The listing builds one solid part. Answer for the finished solid, in the listing's coordinates (mm). A direction names the side the tool comes from. Round coordinates to 2 decimals unless told otherwise and drop trailing zeros. Write each loop counter-clockwise with the first axis right and the second up, starting at its lowest first coordinate (ties: lowest second). Pieces come first, ordered by that corner, then holes.
Item 1: For a pull along Y with two mould halves and no side action, classify faces 1 (the face through (11.01, 6.66, 2.5)), 2 (the face through (6, 2, 4)), 3 (the face through (-3.794, -17.084, 1.479)) as +Y half, -Y half, draft (parallel to the pull), parting line (faces both ways), or undercut.
Item 2: Each of these flat-tipped pins is pushed along its axis until it touches: pin 1 (10.5 mm diameter, centred on x = 12.99, y = -7.5, fed in from +Z); pin 2 (4 mm diameter, centred on y = 3.5, z = 1.5, fed in from +X); pin 3 (6 mm diameter, centred on x = 14, y = -8, fed in from +Z). Where does it stop, or does it pass through?
Item 3: Find section D-D on y = 0. Give the vertices of the cut face in (x, z) (3 decimals).
Item 4: Find the intervals of material crossed by probe 1 along Y at (x, z) = (0, 1); probe 2 along Y at (x, z) = (0, 2.7); probe 3 along Y at (x, z) = (-0.5, 4.75), in increasing order.
Item 5: Find section C-C on z = 5. Give the vertices of the cut face in (x, y) (3 decimals), then the cut area to 3 significant figures.
Item 6: Find section A-A on z = 0.5. Give the vertices of the cut face in (x, y), then the cut area to 3 significant figures.
Item 7: Find section B-B on y = 7.5. Give the vertices of the cut face in (x, z), then the cut area to 3 significant figures.
Item 8: A tool of negligible diameter and unlimited length cuts with its end or side. For faces 4 (the face through (3.476, 0.045, 5.535)), 5 (the face through (-11.083, 8.101, 1.232)), from which of +Z, -Z, +X, -X, +Y, -Y can it reach the whole face along a straight path? Write none if from no direction.
```python
from build123d import *

# Parameters (mm, degrees)
SKETCH_1_R          = 17.5
SKETCH_1_R_2        = 2.5
SKETCH_1_R_3        = 2
EXTRUDE_1_DEPTH     = 3
SKETCH_2_R          = 6
SKETCH_2_R_2        = 2.5
EXTRUDE_2_DEPTH     = 5
SKETCH_4_R          = 4.05
CUT_EXTRUDE_2_DEPTH = 0.5
SKETCH_5_R          = 1.025
CUT_EXTRUDE_3_DEPTH = 5
SKETCH_6_R          = 7
SKETCH_6_R_2        = 5.979713823
EXTRUDE_4_DEPTH     = 1


with BuildPart() as part:
    # 草图1 → 凸台-拉伸1 (new body)
    with BuildSketch(Plane.XY):
        Circle(SKETCH_1_R)
        Circle(SKETCH_1_R_2, mode=Mode.SUBTRACT)
        with Locations((0, 15)):
            Circle(SKETCH_1_R_3, mode=Mode.SUBTRACT)
        with Locations((12.990381057, 7.5)):
            Circle(SKETCH_1_R_3, mode=Mode.SUBTRACT)
        with Locations((12.990381057, -7.5)):
            Circle(SKETCH_1_R_3, mode=Mode.SUBTRACT)
        with Locations((0, -15)):
            Circle(SKETCH_1_R_3, mode=Mode.SUBTRACT)
        with Locations((-12.990381057, -7.5)):
            Circle(SKETCH_1_R_3, mode=Mode.SUBTRACT)
        with Locations((-12.990381057, 7.5)):
            Circle(SKETCH_1_R_3, mode=Mode.SUBTRACT)
    extrude(amount=EXTRUDE_1_DEPTH)

    # 草图2 → 凸台-拉伸2 (add)
    with BuildSketch(Plane.XY.offset(3)):
        Circle(SKETCH_2_R)
        Circle(SKETCH_2_R_2, mode=Mode.SUBTRACT)
    extrude(amount=EXTRUDE_2_DEPTH)

    # 草图4 → 切除-拉伸2 (cut)
    with BuildSketch(Plane.XY.offset(3)):
        with Locations((12.990381057, 7.5)):
            Circle(SKETCH_4_R)
        with Locations((12.990381057, -7.5)):
            Circle(SKETCH_4_R)
        with Locations((0, -15)):
            Circle(SKETCH_4_R)
        with Locations((-12.990381057, -7.5)):
            Circle(SKETCH_4_R)
        with Locations((-12.990381057, 7.5)):
            Circle(SKETCH_4_R)
        with Locations((0, 15)):
            Circle(SKETCH_4_R)
    extrude(amount=-CUT_EXTRUDE_2_DEPTH, mode=Mode.SUBTRACT)

    # 草图5 → 切除-拉伸3 (cut)
    with BuildSketch(Plane.XY.offset(8)):
        with Locations((0, 4.5)):
            Circle(SKETCH_5_R)
        with Locations((4.5, 0)):
            Circle(SKETCH_5_R)
        with Locations((0, -4.5)):
            Circle(SKETCH_5_R)
        with Locations((-4.5, 0)):
            Circle(SKETCH_5_R)
    extrude(amount=-CUT_EXTRUDE_3_DEPTH, mode=Mode.SUBTRACT)

    # 草图6 → 凸台-拉伸4 (add)
    with BuildSketch(Plane.XY.offset(3)):
        Circle(SKETCH_6_R)
        Circle(SKETCH_6_R_2, mode=Mode.SUBTRACT)
    extrude(amount=EXTRUDE_4_DEPTH)


solid = part.part
```
Check values:
1. face 1: undercut
1. face 2: draft
1. face 3: parting line
2. pin 1: stops at z = 3
2. pin 2: stops at x = 17.44
2. pin 3: stops at z = 2.5
3. outline: (-17.5, 0) - (-2.5, 0) - (-2.5, 8) - (-3.475, 8) - (-3.475, 3) - (-5.525, 3) - (-5.525, 8) - (-6, 8) - (-6, 4) - (-7, 4) - (-7, 3) - (-17.5, 3) - close; (2.5, 0) - (17.5, 0) - (17.5, 3) - (7, 3) - (7, 4) - (6, 4) - (6, 8) - (5.525, 8) - (5.525, 3) - (3.475, 3) - (3.475, 8) - (2.5, 8) - close
4. probe 1: y = -17.5 to -17, -13 to -2.5, 2.5 to 13, 17 to 17.5
4. probe 2: y = -10.95 to -2.5, 2.5 to 10.95
4. probe 3: y = -5.98 to -5.39, -3.61 to -2.45, 2.45 to 3.61, 5.39 to 5.98
5. outline: circle Ø12 at (0, 0); hole circle Ø2.05 at (-4.5, 0); hole circle Ø5 at (0, 0); hole circle Ø2.05 at (0, -4.5); hole circle Ø2.05 at (0, 4.5); hole circle Ø2.05 at (4.5, 0)
5. area: 80.3 mm2
6. outline: circle Ø35 at (0, 0); hole circle Ø4 at (-12.99, -7.5); hole circle Ø4 at (-12.99, 7.5); hole circle Ø5 at (0, 0); hole circle Ø4 at (0, -15); hole circle Ø4 at (0, 15); hole circle Ø4 at (12.99, -7.5); hole circle Ø4 at (12.99, 7.5)
6. area: 867 mm2
7. outline: (-15.81, 0) - (-14.99, 0) - (-14.99, 2.5) - (-15.81, 2.5) - close; (-10.99, 0) - (10.99, 0) - (10.99, 2.5) - (8.94, 2.5) - (8.94, 3) - (-8.94, 3) - (-8.94, 2.5) - (-10.99, 2.5) - close; (14.99, 0) - (15.81, 0) - (15.81, 2.5) - (14.99, 2.5) - close
7. area: 68.0 mm2
8. face 4: +Z
8. face 5: +Z, -Z
